Input: part model. Units: mm. Frame: model coordinates. Face numbers are marked on the shaded views. A direction names the side the tool comes from. Round coordinates to 2 decimals unless told otherwise and drop trailing zeros. Order: outer loops, then holes, each group sorted by start corner. A loop starts at its lowest first (then second) coordinate and runs counter-clockwise, first axis right, second up. Notation, with made-up numbers: (-3.5, 46.25) - (24.5, 46.25) arc R25 cw to (24.5, 68.25) - close; hole circle Ø9 at (29, 35). An arc over 180 degrees is marked (long way). One line per item, written item: value. Start each with the question number.
from build123d import *

# Parameters (mm, degrees)
SKETCH_1_W          = 20
SKETCH_1_H          = 20
EXTRUDE_1_DEPTH     = 20
EXTRUDE_1_2_DEPTH   = 20
SKETCH_1_3_W        = 20
SKETCH_1_3_H        = 20
EXTRUDE_2_DEPTH     = 40
EXTRUDE_3_DEPTH     = 5
SKETCH_3_W          = 5
SKETCH_3_H          = 40
EXTRUDE_4_DEPTH     = 5
SKETCH_5_W          = 40
SKETCH_5_H          = 5
EXTRUDE_5_DEPTH     = 5
SKETCH_6_W          = 15
SKETCH_6_H          = 15
CUT_EXTRUDE_1_DEPTH = 40
SKETCH_7_R          = 2.5
CUT_EXTRUDE_2_DEPTH = 5
SKETCH_9_R          = 2.5
CUT_EXTRUDE_3_DEPTH = 5
SKETCH_10_R         = 2.5
CUT_EXTRUDE_4_DEPTH = 5
FILLET_1_R          = 3


with BuildPart() as part:
    # Sketch 1 → Extrude 1 (new body)
    with BuildSketch(Plane(origin=(0, 0, 0), x_dir=(1, 0, 0), z_dir=(0, 1, 0))):
        with Locations((10, 30)):
            Rectangle(SKETCH_1_W, SKETCH_1_H)
    extrude(amount=EXTRUDE_1_DEPTH)



with BuildPart() as body_2:
    # Sketch 1 → Extrude 1 2 (new body)
    with BuildSketch(Plane(origin=(0, 0, 0), x_dir=(1, 0, 0), z_dir=(0, 1, 0))):
        with Locations((30, 10)):
            Rectangle(SKETCH_1_W, SKETCH_1_H)
    extrude(amount=EXTRUDE_1_2_DEPTH)


with BuildPart() as part_1:
    add(part.part)

    add(body_2.part)  # Extrude 2 merges body 2
    # Sketch 1_3 → Extrude 2 (add)
    with BuildSketch(Plane(origin=(0, 0, 0), x_dir=(1, 0, 0), z_dir=(0, 1, 0))):
        with Locations((10, 10)):
            Rectangle(SKETCH_1_3_W, SKETCH_1_3_H)
    extrude(amount=EXTRUDE_2_DEPTH)



with BuildPart() as body_2_2:
    # Sketch 2 → Extrude 3 (new body)
    with BuildSketch(Plane.XY):
        Polygon((0, 0), (40, 0), (40, 20), (20, 20), (20, 40), (0, 40), align=None)
    extrude(amount=EXTRUDE_3_DEPTH)


with BuildPart() as body_3:
    # Sketch 3 → Extrude 4 (new body)
    with BuildSketch(Plane.ZY):
        Polygon((-20, 20), (-40, 20), (-40, 0), (0, 0), (0, 40), (-20, 40), align=None)
        with Locations((2.5, 20)):
            Rectangle(SKETCH_3_W, SKETCH_3_H)
    extrude(amount=EXTRUDE_4_DEPTH)


with BuildPart() as part_2:
    add(part_1.part)

    add(body_2_2.part)  # Extrude 5 merges body 2 2

    add(body_3.part)  # Extrude 5 merges body 3
    # Sketch 5 → Extrude 5 (add)
    with BuildSketch(Plane.XZ):
        with Locations((20, 2.5)):
            Rectangle(SKETCH_5_W, SKETCH_5_H)
        Polygon((0, 0), (0, -40), (20, -40), (20, -20), (40, -20), (40, 0), align=None)
        Polygon((-5, 5), (-5, -40), (0, -40), (0, 0), (0, 5), align=None)
    extrude(amount=EXTRUDE_5_DEPTH)

    # Sketch 6 → Cut-Extrude 1 (cut)
    with BuildSketch(Plane(origin=(0, 40, 0), x_dir=(1, 0, 0), z_dir=(0, 1, 0))):
        Polygon((0, 0), (20, 0), (20, 15), (20, 20), (15, 20), (0, 20), align=None)
        with Locations((7.5, 27.5)):
            Rectangle(SKETCH_6_W, SKETCH_6_H)
        Polygon((15, 20), (20, 20), (20, 40), (0, 40), (0, 35), (15, 35), align=None)
        with Locations((27.5, 7.5)):
            Rectangle(SKETCH_6_W, SKETCH_6_H)
        Polygon((20, 20), (20, 15), (35, 15), (35, 0), (40, 0), (40, 20), align=None)
    extrude(amount=-CUT_EXTRUDE_1_DEPTH, mode=Mode.SUBTRACT)

    # Sketch 7 → Cut-Extrude 2 (cut)
    with BuildSketch(Plane(origin=(0, 0, 0), x_dir=(1, 0, 0), z_dir=(0, 1, 0))):
        with Locations(Location((10, 30, 0), (0, 0, 270))):
            Circle(SKETCH_7_R)
        with Locations(Location((30, 10, 0), (0, 0, 270))):
            Circle(SKETCH_7_R)
        with Locations(Location((10, 10, 0), (0, 0, 270))):
            Circle(SKETCH_7_R)
    extrude(amount=-CUT_EXTRUDE_2_DEPTH, mode=Mode.SUBTRACT)

    # Sketch 9 → Cut-Extrude 3 (cut)
    with BuildSketch(Plane(origin=(0, 0, 0), x_dir=(-1, 0, 0), z_dir=(0, 0, -1))):
        with Locations((-10, 30)):
            Circle(SKETCH_9_R)
        with Locations((-30, 10)):
            Circle(SKETCH_9_R)
        with Locations((-10, 10)):
            Circle(SKETCH_9_R)
    extrude(amount=-CUT_EXTRUDE_3_DEPTH, mode=Mode.SUBTRACT)

    # Sketch 10 → Cut-Extrude 4 (cut)
    with BuildSketch(Plane(origin=(0, 0, 0), x_dir=(0, 0, -1), z_dir=(1, 0, 0))):
        with Locations((10, 30)):
            Circle(SKETCH_10_R)
        with Locations((30, 10)):
            Circle(SKETCH_10_R)
        with Locations((10, 10)):
            Circle(SKETCH_10_R)
    extrude(amount=-CUT_EXTRUDE_4_DEPTH, mode=Mode.SUBTRACT)

    # Fillet 1
    fillet_1_edges = [part_2.edges().sort_by_distance(p)[0] for p in [
        (-5, 17.5, 5),
        (-5, 7.5, -40),
        (40, 7.5, 5),
        (-5, -5, -17.5),
        (7.5, -5, -40),
        (40, -5, -7.5),
        (17.5, -5, 5),
        (7.5, 40, 5),
        (-5, 40, -7.5),
    ]]
    fillet(fillet_1_edges, radius=FILLET_1_R)


solid = part_2.part
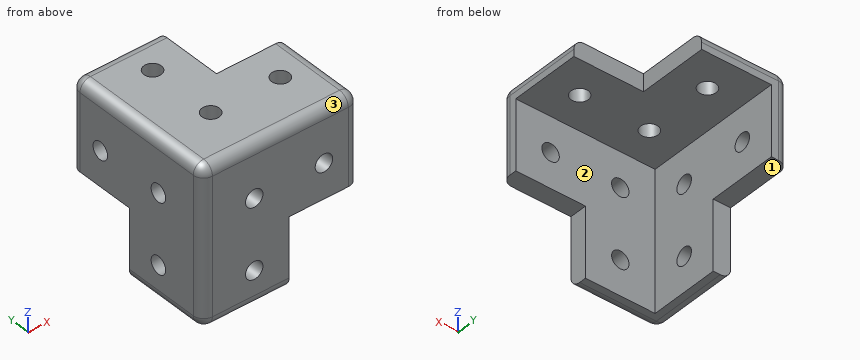
Item 1: Line query: L1, parallel to Y at x = -2.3, z = -10; L2, parallel to X at y = 19, z = -30.5; L3, parallel to Z at x = 36.5, y = 1.5. Output: solid intervals per line, ascending.
Item 2: Section query A-A on z = -30. Return loops of the section in (x, y).
Item 3: Section query C-C on y = 10. Return loops of the section in (x, z).
Item 4: Reachability of the marked faces 1, 2 and 3 from +Z, -Z, +X, -X, +Y, -Y: full face, straight path, thin tool, end or side. Return the list, or none.
Item 5: First-contact query: pin 1 Ø6 at (y, z) = (9.5, -24.5) entering from +X; pin 2 Ø6 at (x, z) = (10, -10) entering from -Y; pin 3 Ø1.5 at (x, y) = (22.5, 31.5) entering from -Z; pin 4 Ø1.5 at (y, z) = (25.5, 3.5) entering from +X. Flat tips, straight axial feed; report the tip coordinate or a pass-through.
Item 6: Section query B-B on x = 28.5. Return loops of the section in (y, z), and give its area (3 significant figures).
Geometry results:
1. L1: y = -4.98 to 7.5, 12.5 to 27.5, 32.5 to 39.98
1. L2: x = -5 to 0
1. L3: z = 0 to 5
2. outline: (-5, -2) arc R3 ccw to (-2, -5) - (7.5, -5) - (7.5, 0) - (0, 0) - (0, 7.5) - (-5, 7.5) - close; (-5, 12.5) - (0, 12.5) - (0, 20) - (-5, 20) - close; (12.5, -5) - (20, -5) - (20, 0) - (12.5, 0) - close
3. outline: (-5, -37) arc R3 ccw to (-2, -40) - (0, -40) - (0, -32.5) - (-5, -32.5) - close; (-5, -27.5) - (0, -27.5) - (0, -12.5) - (-5, -12.5) - close; (-5, -7.5) - (0, -7.5) - (0, 0) - (7.5, 0) - (7.5, 5) - (-2, 5) arc R3 ccw to (-5, 2) - close; (12.5, 0) - (27.5, 0) - (27.5, 5) - (12.5, 5) - close; (32.5, 0) - (40, 0) - (40, 2) arc R3 ccw to (37, 5) - (32.5, 5) - close
4. face 1: -Z, +X, -X, +Y
4. face 2: -Z, +X, +Y
4. face 3: +Z, +X, -X, -Y
5. pin 1: stops at x = 0
5. pin 2: stops at y = -5
5. pin 3: passes through
5. pin 4: stops at x = 20
6. outline: (-5, -20) - (0, -20) - (0, -12) - (-5, -12) - close; (-5, -8) - (0, -8) - (0, 0) - (8, 0) - (8, 5) - (-2, 5) arc R3 ccw to (-5, 2) - close; (12, 0) - (20, 0) - (20, 5) - (12, 5) - close
6. area: 183 mm^2
